```python
from build123d import *

# Parameters (mm, degrees)
BOSS_EXTRUDE1_DEPTH      = 40
F_1_0_1_DIAMETER_HOLE1_D = 85
SKETCH8_R                = 50
BOSS_EXTRUDE2_DEPTH      = 250
FILLET1_R                = 50
CHAMFER1_SIZE            = 50


with BuildPart() as part:
    # Sketch1 → Boss-Extrude1 (new body)
    with BuildSketch(Plane(origin=(0, 0, 0), x_dir=(1, 0, 0), z_dir=(0, 1, 0))):
        Polygon((-65.68627451, 1095.876515785), (754.006770172, -323.873484215), (-885.379319192, -323.873484215), align=None)
    extrude(amount=BOSS_EXTRUDE1_DEPTH)

    # Ø1.0 (1) Diameter Hole1 (through all)
    with Locations(Plane(origin=(0, 40, 0), x_dir=(1, 0, 0), z_dir=(0, 1, 0))):
        with Locations((-65.68627451, 975.876515785), (-781.456270738, -263.873484215), (650.083721718, -263.873484215)):
            Hole(F_1_0_1_DIAMETER_HOLE1_D / 2)

    # Sketch8 → Boss-Extrude2 (add)
    with BuildSketch(Plane(origin=(0, 0, 0), x_dir=(-1, 0, 0), z_dir=(0, -1, 0))):
        with Locations(Location((65.68627451, 149.376515785, 0), (0, 0, 90))):
            Circle(SKETCH8_R)
    extrude(amount=-BOSS_EXTRUDE2_DEPTH)

    # Fillet1
    fillet1_edges = [part.edges().sort_by_distance(p)[0] for p in [
        (-885.379319192, 20, 323.873484215),
        (754.006770172, 20, 323.873484215),
        (-65.68627451, 20, -1095.876515785),
    ]]
    fillet(fillet1_edges, radius=FILLET1_R)

    # Chamfer1
    chamfer1_edges = [part.edges().sort_by_distance(p)[0] for p in [
        (-65.68627451, 250, -99.376515785),
    ]]
    chamfer(chamfer1_edges, length=CHAMFER1_SIZE)


solid = part.part
```
Check sheet for the modelled part. Datum: model origin and axes. Units: mm. A direction names the side the tool comes from. Coordinates: 2 decimals unless noted, no trailing zeros. Order: outer loops, then holes, each group sorted by start corner. A loop starts at its lowest first (then second) coordinate and runs counter-clockwise, first axis right, second up. Notation, with made-up numbers: M -20,8.5 L 9,8.5 A14 ccw 9,16.5 Z; hole C 8.25,-9.5 d8. An arc over 180 degrees is marked long. Write each question's results on one line, items separated by ' | '. Start each with the question number.
1. Go/stop test with a flat-tipped pin: P1, Ø3, axis at x = -393, z = 165.5, coming from the +Y side. Record where the tip stops, or that it passes through.
2. Cross-section at A-A on z = -589.5. Record the cut outline in (x, y).
3. Material ranges on probe 1 along Y at (x, z) = (270, 208); probe 2 along Z at (x, y) = (16, 30); probe 3 along Z at (x, y) = (301, 31), recorded low to high.
4. Mould release check, pull along X, two halves, no side actions. Record for faces 1 (the face through (-64.95, 20.28, -1045.87)), 2 (the face through (-56.473, 19.72, -934.387)), 3 (the face through (339.03, 19.72, -394.89)), 4 (the face through (-820.715, 19.72, 280.151)): +X half, -X half, draft (parallel to the pull), parting line (faces both ways), or undercut.
5. Cross-section at C-C on y = 154. Record the cut outline in (x, z), and give its area (3 significant figures).
6. Cross-section at B-B on x = -626.5. Record the cut outline in (y, z), and give its area (3 significant figures).
7. Access from +Z, -Z, +X, -X, +Y, -Y to the whole of each face (thin tool, end or side, straight path). Record for faces 5 (the face through (-31.894, 118.88, -112.524)), 6 (the face through (-842.44, 20.28, 298.236)).
Checks:
1) P1: stops at y = 40
2) outline: M -358.04,0 L 226.67,0 L 226.67,40 L -358.04,40 Z
3) probe 1: y = 0 to 40 | probe 2: z = -954.39 to 323.87 | probe 3: z = -460.76 to 323.87
4) face 1: parting line | face 2: undercut | face 3: +X half | face 4: undercut
5) outline: C -65.69,-149.38 d100 | area: 7,850 mm²
6) outline: M 0,-124.52 L 40,-124.52 L 40,323.87 L 0,323.87 Z | area: 17,900 mm²
7) face 5: +Y | face 6: -X, +Y, -Y
